Design review of the part built by this model. Coordinates are the model's own, in mm. A direction names the side the tool comes from. Coordinates: 2 decimals unless noted, no trailing zeros. Write each loop counter-clockwise with the first axis right and the second up, starting at its lowest first coordinate (ties: lowest second). Pieces come first, ordered by that corner, then holes.
Q1. The part is to be moulded in two halves that separate along X. For faces 5 (the face through (7.5, 15, 2)), 6 (the face through (-38.61, 16.41, 0.79)), 7 (the face through (-35.75, -1, 5)), say which applies: +X half, -X half, draft (parallel to the pull), parting line (faces both ways), or undercut.
Q2. To check wall thickness, follow probe 1 along Y at (x, z) = (37.5, 1.25); probe 2 along Y at (x, z) = (28.5, 4.75); probe 3 along Z at (x, y) = (-10.5, 7.5). State the ranges of each line that lie inside material, in increasing order.
Q3. Add section A-A, the plane y = 15.4. Give the boundary of the cut face in (x, z), plus the area to 3 significant figures.
Q4. Add section D-D, the plane x = 28. Give the boundary of the cut face in (y, z), plus the area to 3 significant figures.
Q5. Clearance check with flat-ended pins moving along their axes: pin 1 Ø4 at (x, z) = (-8.5, -3.5) entering from +Y; pin 2 Ø7.5 at (x, z) = (-7.5, 6.5) entering from -Y; pin 3 Ø3.5 at (x, y) = (-37.5, 15.4) entering from +Z; pin 4 Ø1.5 at (y, z) = (15.5, 2) entering from -X. State where each tip first meets the part, or that it passes through.
Q6. Machinability: for faces 1 (the face through (-13, 14.1, -4)), 2 (the face through (-13, 14.1, 2)), 3 (the face through (-13, 15, 3)), 4 (the face through (-1, -12.8, 5)), which of the approach directions +Z, -Z, +X, -X, +Y, -Y give a long, thin tool a straight path to every point of the face, cutting with its end or side? Answer none if there is none.
Q7. Add section C-C, the plane y = 0. Give the boundary of the cut face in (x, z), plus the area to 3 significant figures.
Q8. Add section B-B, the plane x = -37.5. Give the boundary of the cut face in (y, z).
from build123d import *

# Parameters (mm, degrees)
F0_R          = 1.5
F0_W          = 40.7
F0_H          = 2.6
F1_DEPTH      = 1.6
F2_DEPTH      = 8.64
F3_DEPTH      = 8.4
F3_DEPTH_BACK = 3
F4_DEPTH      = 4.5


with BuildPart() as f1:
    # F0 (on Top) → F1 (new body)
    with BuildSketch(Plane.XY):
        Polygon((40, 18.1), (-40, 18.1), (-40, -18.1), (40, -18.1), (40, -2.475), (35.35, -7.8), (35.35, -12.8), (-35.75, -12.8), (-35.75, 11.35), (35.35, 11.35), (35.35, 6.35), (40, 1.025), align=None)
        with Locations((-37.5, -15.5)):
            Circle(F0_R, mode=Mode.SUBTRACT)
        with Locations((37.5, -15.5)):
            Circle(F0_R, mode=Mode.SUBTRACT)
        with Locations((-37.5, 15.4)):
            Circle(F0_R, mode=Mode.SUBTRACT)
        with Locations((-12.85, 15.4)):
            Rectangle(F0_W, F0_H, mode=Mode.SUBTRACT)
        with Locations((37.5, 15.4)):
            Circle(F0_R, mode=Mode.SUBTRACT)
        Polygon((35.35, -7.8), (35.35, 6.35), (35.35, 11.35), (-35.75, 11.35), (-35.75, -12.8), (35.35, -12.8), align=None)
    extrude(amount=F1_DEPTH)

    # F0 (on Top) → F2 (join)
    with BuildSketch(Plane.XY):
        Polygon((35.35, -7.8), (35.35, 6.35), (35.35, 11.35), (-35.75, 11.35), (-35.75, -12.8), (35.35, -12.8), align=None)
    extrude(amount=F2_DEPTH)

    # F0 (on Top) → F3 (join, two sides)
    with BuildSketch(Plane.XY) as f3_sk:
        with Locations((-12.85, 15.4)):
            Rectangle(F0_W, F0_H)
    extrude(amount=-F3_DEPTH)
    extrude(f3_sk.sketch, amount=F3_DEPTH_BACK)

    # F0 (on Top) → F4 (join)
    with BuildSketch(Plane.XY):
        Polygon((40, -2.475), (40, 1.025), (35.35, 6.35), (35.35, -7.8), align=None)
    extrude(amount=F4_DEPTH)


solid = f1.part
Here are the results:
1. face 5: +X half
1. face 6: undercut
1. face 7: -X half
2. probe 1: y = -18.1 to -17, -14 to 13.9, 16.9 to 18.1
2. probe 2: y = -12.8 to 11.35
2. probe 3: z = 0 to 8.64
3. outline: (-40, 0) - (-39, 0) - (-39, 1.6) - (-40, 1.6) - close; (-36, 0) - (-33.2, 0) - (-33.2, -8.4) - (7.5, -8.4) - (7.5, 0) - (36, 0) - (36, 1.6) - (7.5, 1.6) - (7.5, 3) - (-33.2, 3) - (-33.2, 1.6) - (-36, 1.6) - close; (39, 0) - (40, 0) - (40, 1.6) - (39, 1.6) - close
3. area: 517 mm2
4. outline: (-18.1, 0) - (18.1, 0) - (18.1, 1.6) - (11.35, 1.6) - (11.35, 8.64) - (-12.8, 8.64) - (-12.8, 1.6) - (-18.1, 1.6) - close
4. area: 228 mm2
5. pin 1: stops at y = 16.7
5. pin 2: stops at y = -12.8
5. pin 3: stops at z = 1.6
5. pin 4: stops at x = -40
6. face 1: -Z, +X, -X, -Y
6. face 2: +Z, +X, -X
6. face 3: +Z, +X, -X, +Y
6. face 4: +Z, +X, -X, -Y
7. outline: (-40, 0) - (40, 0) - (40, 4.5) - (35.35, 4.5) - (35.35, 8.64) - (-35.75, 8.64) - (-35.75, 1.6) - (-40, 1.6) - close
7. area: 642 mm2
8. outline: (-18.1, 0) - (-17, 0) - (-17, 1.6) - (-18.1, 1.6) - close; (-14, 0) - (13.9, 0) - (13.9, 1.6) - (-14, 1.6) - close; (16.9, 0) - (18.1, 0) - (18.1, 1.6) - (16.9, 1.6) - close
